Can you work these out from the model? Positions are in its coordinate system, mm. Round coordinates to 2 decimals unless told otherwise and drop trailing zeros. Loops run counter-clockwise (first coordinate to the right, second up) from the corner with the lowest first, then second, coordinate; pieces in that order, holes last. Notation, with made-up numbers: M 7.25,68 L 26.25,68 A23 ccw 26.25,89 Z; hole C -20,-24 d6. An arc over 180 degrees is marked long. Return JSON: item names as keys, results as strings.
```python
from build123d import *

# Parameters (mm, degrees)
F0_R     = 2
F1_DEPTH = 5.5


with BuildPart() as f1:
    # F0 (on Front) → F1 (new body)
    with BuildSketch(Plane.XZ):
        with BuildLine():
            ThreePointArc((-12.028302, -2.911898), (0, -1.443537), (12.028302, -2.911898))
            ThreePointArc((12.028302, -2.911898), (15.75, 0), (12.028302, 2.911898))
            ThreePointArc((12.028302, 2.911898), (0, 1.443537), (-12.028302, 2.911898))
            ThreePointArc((-12.028302, 2.911898), (-15.75, 0), (-12.028302, -2.911898))
        make_face()
        with Locations((-12.75, 0)):
            Circle(F0_R, mode=Mode.SUBTRACT)
        with Locations((12.75, 0)):
            Circle(F0_R, mode=Mode.SUBTRACT)
    extrude(amount=F1_DEPTH)


solid = f1.part
```
Q1. If I drill on line 1 along X through (y, z) = (-3.45, 0.1); line 2 along Z through (x, y) = (12.75, -4.3); line 3 along Z through (x, y) = (-12, -1.2), over which ranges is the centre line in solid material (lowest first)?
Results:
{"line 1": "x = -15.75 to -14.75, -10.75 to 10.75, 14.75 to 15.75", "line 2": "z = -3 to -2, 2 to 3", "line 3": "z = -2.9 to -1.85, 1.85 to 2.9"}
Q2. Suppose I cut it at B-B, the plane z = 0. Please give me the cut outline in (x, y).
Results:
{"outline": "M -15.75,-5.5 L -14.75,-5.5 L -14.75,0 L -15.75,0 Z; M -10.75,-5.5 L 10.75,-5.5 L 10.75,0 L -10.75,0 Z; M 14.75,-5.5 L 15.75,-5.5 L 15.75,0 L 14.75,0 Z"}
Q3. Suppose I cut it at C-C, the plane z = 2.6. Please give me the cut outline in (x, y), plus the area to 3 significant figures.
Results:
{"outline": "M -14.25,-5.5 L -10.69,-5.5 L -10.69,0 L -14.25,0 Z; M 10.69,-5.5 L 14.25,-5.5 L 14.25,0 L 10.69,0 Z", "area": "39.1 mm2"}
Q4. Suppose I cut it at D-D, the plane y = -0.55. Please give me the cut outline in (x, z), plus the area to 3 significant figures.
Results:
{"outline": "M -12.03,-2.91 A50 cw 12.03,-2.91 A3 ccw long 12.03,2.91 A50 cw -12.03,2.91 A3 ccw long Z; hole C -12.75,0 d4; hole C 12.75,0 d4", "area": "105 mm2"}
Q5. Suppose I cut it at A-A, the plane x = 12.75. Please give me the cut outline in (y, z).
Results:
{"outline": "M -5.5,-3 L 0,-3 L 0,-2 L -5.5,-2 Z; M -5.5,2 L 0,2 L 0,3 L -5.5,3 Z"}
Q6. Thinking about a two-plate mould opening in Z: for faces 1 (the cylindrical face through (-14.337, -2.712, -1.217)), 2 (the cylindrical face through (-0.17, -2.712, -1.444)), 3 (the cylindrical face through (15.75, -2.71, -0.08)), which applies, pulls with the +Z half, pulls with the -Z half, needs draft (parallel to the pull), parting line crosses it, or undercut?
Results:
{"face 1": "undercut", "face 2": "pulls with the -Z half", "face 3": "parting line crosses it"}
Q7. I'm going to push a flat-ended pin straight in: pin 1 Ø1 at (y, z) = (-4, 0.5) entering from +X. Where does the tip first touch, or does it pass through?
Results:
{"pin 1": "stops at x = 15.75"}
